```python
from build123d import *

# Parameters (mm, degrees)
SKETCH1_W           = 42.3
SKETCH1_H           = 5
BOSS_EXTRUDE1_DEPTH = 4
CHAMFER1_SIZE       = 5


with BuildPart() as part:
    # Sketch1 → Boss-Extrude1 (new body)
    with BuildSketch(Plane.YZ):
        Polygon((-21.921641791, 5.223880597), (-17.921641791, 5.223880597), (24.378358209, 5.223880597), (66.678358209, 5.223880597), (70.678358209, 5.223880597), (70.678358209, 0.223880597), (75.678358209, 0.223880597), (75.678358209, 12.723880597), (-26.921641791, 12.723880597), (-26.921641791, 0.223880597), (-21.921641791, 0.223880597), align=None)
        with Locations((3.228358209, 2.723880597)):
            Rectangle(SKETCH1_W, SKETCH1_H)
        with Locations((45.528358209, 2.723880597)):
            Rectangle(SKETCH1_W, SKETCH1_H)
    extrude(amount=BOSS_EXTRUDE1_DEPTH)

    # Chamfer1
    chamfer1_edges = [part.edges().sort_by_distance(p)[0] for p in [
        (2, -26.921641791, 12.723880597),
        (2, 75.678358209, 12.723880597),
    ]]
    chamfer(chamfer1_edges, length=CHAMFER1_SIZE)


solid = part.part
```
Could you check a few things on this model? Use its own coordinates, in mm. A direction names the side the tool comes from. Give positions to 0.01 mm unless a question says otherwise; leave off trailing zeros. Loops run counter-clockwise (first coordinate to the right, second up) from the corner with the lowest first, then second, coordinate; pieces in that order, holes last. Notation, with made-up numbers: (49.5, -35.75) - (60.5, -35.75) arc R15 ccw to (60.5, -19.75) - close; hole circle Ø4 at (-26.5, -18.5). An arc over 180 degrees is marked (long way). Use one line per item in the form item = value.
1. I want a section at B-B (x = 1.15). Please give me the cut outline in (y, z).
Response values:
outline = (-26.92, 0.22) - (-21.92, 0.22) - (-21.92, 5.22) - (-17.92, 5.22) - (-17.92, 0.22) - (66.68, 0.22) - (66.68, 5.22) - (70.68, 5.22) - (70.68, 0.22) - (75.68, 0.22) - (75.68, 7.72) - (70.68, 12.72) - (-21.92, 12.72) - (-26.92, 7.72) - close
2. I need wall thicknesses on probe 1 along Y at (x, z) = (1.6, 4.25); probe 2 along Z at (x, y) = (0.4, -20); probe 3 along Y at (x, z) = (0.5, 8). Which ranges of each line are inside material? Lowest first, please.
Response values:
probe_1 = -26.92 to -21.92, -17.92 to 66.68, 70.68 to 75.68
probe_2 = 5.22 to 12.72
probe_3 = -26.65 to 75.4
3. I'm going to push flat-ended pins straight in: pin 1 Ø2 at (x, y) = (1.5, -20) entering from -Z; pin 2 Ø1 at (x, z) = (3, 10) entering from -Y. Where does each tip first touch, or does it pass through?
Response values:
pin_1 = 5.22
pin_2 = -25.15
4. On a 3-axis mill with a long thin cutter (end or side, diameter ignored), from which of +Z, -Z, +X, -X, +Y, -Y can I reach the whole of each face in a straight line? I mean faces 1 (the face through (4, 24, 7)), 2 (the face through (2, -17.922, 3)). Say none if no direction works.
Response values:
face_1 = +Z, -Z, +X, +Y, -Y
face_2 = -Z, +X, -X
5. Thinking about a two-plate mould opening in Y: for faces 3 (the face through (2, 66.678, 3)), 4 (the face through (2, 73.1, 10.3)), 5 (the face through (2, 73, 0.224)), 6 (the face through (2, -21.922, 3)), which applies, released by +Y, released by -Y, zero draft, split by the parting line, or undercut?
Response values:
face_3 = undercut
face_4 = released by +Y
face_5 = zero draft
face_6 = undercut
6. I want a section at A-A (z = 2.25). Please give me the cut outline in (x, y).
Response values:
outline = (0, -26.92) - (4, -26.92) - (4, -21.92) - (0, -21.92) - close; (0, -17.92) - (4, -17.92) - (4, 66.68) - (0, 66.68) - close; (0, 70.68) - (4, 70.68) - (4, 75.68) - (0, 75.68) - close
